Verification items for the finished model (mm, model axes). A direction names the side the tool comes from. Give positions to 0.01 mm unless a question says otherwise; leave off trailing zeros. Write each loop counter-clockwise with the first axis right and the second up, starting at its lowest first coordinate (ties: lowest second). Pieces come first, ordered by that corner, then holes. Notation, with made-up numbers: (-13.75, 69.5) -> (-7.75, 69.5) arc R33 cw to (-7.75, 107.5) -> close; hole circle Ø11 at (72.5, 82.25). An arc over 180 degrees is marked (long way). Write item = value, one per line.
from build123d import *

# Parameters (mm, degrees)
BOSS_EXTRUDE1_DEPTH = 12.7
BOSS_EXTRUDE3_DEPTH = 12.7
CUT_EXTRUDE1_REACH  = 14.7
CUT_EXTRUDE2_REACH  = 14.7
SKETCH6_W           = 7.112
SKETCH6_H           = 3.302
BOSS_EXTRUDE4_DEPTH = 3.175
SKETCH7_W           = 7.112
SKETCH7_H           = 3.302
BOSS_EXTRUDE5_DEPTH = 3.175
CUT_EXTRUDE3_REACH  = 14.7
SKETCH8_W           = 7.112
SKETCH8_H           = 3.302
CUT_EXTRUDE4_REACH  = 14.7
SKETCH9_W           = 7.112
SKETCH9_H           = 3.302


with BuildPart() as part:
    # Sketch1 → Boss-Extrude1 (new body)
    with BuildSketch(Plane(origin=(0, 0, 0), x_dir=(0, 0, -1), z_dir=(1, 0, 0))):
        Polygon((0, 0), (80.01, 0), (80.01, 19.05), (71.12, 19.05), (71.12, 8.89), (8.89, 8.89), (8.89, 19.05), (0, 19.05), align=None)
    extrude(amount=BOSS_EXTRUDE1_DEPTH)

    # Sketch2 → Boss-Extrude3 (add)
    with BuildSketch(Plane.ZY):
        Polygon((-63.5, 12.192), (-70.612, 12.192), (-70.612, 8.89), (-74.93, 8.89), (-74.93, 15.494), (-63.5, 15.494), align=None)
        Polygon((-16.51, 12.192), (-9.398, 12.192), (-9.398, 8.89), (-5.08, 8.89), (-5.08, 15.494), (-16.51, 15.494), align=None)
    extrude(amount=-BOSS_EXTRUDE3_DEPTH)

    # Sketch4 → Cut-Extrude1 (cut, up to next)
    with BuildSketch(Plane.ZY, mode=Mode.PRIVATE) as cut_extrude1_sk1:
        Polygon((-71.12, 15.494), (-75.438, 15.494), (-75.438, 0), (-80.01, 0), (-80.01, 19.05), (-71.12, 19.05), align=None)
    cut_extrude1_tool1 = extrude(cut_extrude1_sk1.sketch, amount=-CUT_EXTRUDE1_REACH, mode=Mode.PRIVATE) & part.part
    add(cut_extrude1_tool1.solids().sort_by_distance((0, 10.686074, -77.05781))[0], mode=Mode.SUBTRACT)

    # Sketch5 → Cut-Extrude2 (cut, up to next)
    with BuildSketch(Plane.ZY, mode=Mode.PRIVATE) as cut_extrude2_sk1:
        Polygon((-8.89, 15.494), (-4.572, 15.494), (-4.572, 0), (0, 0), (0, 19.05), (-8.89, 19.05), align=None)
    cut_extrude2_tool1 = extrude(cut_extrude2_sk1.sketch, amount=-CUT_EXTRUDE2_REACH, mode=Mode.PRIVATE) & part.part
    add(cut_extrude2_tool1.solids().sort_by_distance((0, 10.686074, -2.95219))[0], mode=Mode.SUBTRACT)

    # Sketch6 → Boss-Extrude4 (add)
    with BuildSketch(Plane(origin=(12.7, 0, 0), x_dir=(0, 0, -1), z_dir=(1, 0, 0))):
        with Locations((12.954, 10.541)):
            Rectangle(SKETCH6_W, SKETCH6_H)
    extrude(amount=-BOSS_EXTRUDE4_DEPTH)

    # Sketch7 → Boss-Extrude5 (add)
    with BuildSketch(Plane(origin=(12.7, 0, 0), x_dir=(0, 0, -1), z_dir=(1, 0, 0))):
        with Locations((67.056, 10.541)):
            Rectangle(SKETCH7_W, SKETCH7_H)
    extrude(amount=-BOSS_EXTRUDE5_DEPTH)

    # Sketch8 → Cut-Extrude3 (cut, up to next)
    with BuildSketch(Plane(origin=(12.7, 0, 0), x_dir=(0, 0, -1), z_dir=(1, 0, 0)), mode=Mode.PRIVATE) as cut_extrude3_sk1:
        with Locations((12.954, 10.541)):
            Rectangle(SKETCH8_W, SKETCH8_H)
    cut_extrude3_tool1 = extrude(cut_extrude3_sk1.sketch, amount=-CUT_EXTRUDE3_REACH, mode=Mode.PRIVATE) & part.part
    add(cut_extrude3_tool1.solids().sort_by_distance((12.7, 10.541, -12.954))[0], mode=Mode.SUBTRACT)

    # Sketch9 → Cut-Extrude4 (cut, up to next)
    with BuildSketch(Plane(origin=(12.7, 0, 0), x_dir=(0, 0, -1), z_dir=(1, 0, 0)), mode=Mode.PRIVATE) as cut_extrude4_sk1:
        with Locations((67.056, 10.541)):
            Rectangle(SKETCH9_W, SKETCH9_H)
    cut_extrude4_tool1 = extrude(cut_extrude4_sk1.sketch, amount=-CUT_EXTRUDE4_REACH, mode=Mode.PRIVATE) & part.part
    add(cut_extrude4_tool1.solids().sort_by_distance((12.7, 10.541, -67.056))[0], mode=Mode.SUBTRACT)


solid = part.part
Item 1: Sectioned sample at A-A on y = 10.25. Record the cut outline in (x, z), then the cut area to 3 significant figures.
Response values:
outline = (0, -75.44) -> (12.7, -75.44) -> (12.7, -70.61) -> (0, -70.61) -> close; (0, -9.4) -> (12.7, -9.4) -> (12.7, -4.57) -> (0, -4.57) -> close
area = 123 mm^2
Item 2: Mould release check, pull along Y, two halves, no side actions. Record for faces 4 (the flat face through (12.7, 6, -40)), 5 (the flat face through (6, 15.494, -70)), 6 (the flat face through (6, 8.89, -40)): +Y half, -Y half, draft (parallel to the pull), parting line (faces both ways), or undercut.
Response values:
face_4 = draft
face_5 = +Y half
face_6 = undercut
Item 3: Material ranges on line 1 (Z direction, x = 7.5, y = 14.25); line 2 (Z direction, x = 4.5, y = 11); line 3 (Y direction, x = 5.75, z = -14.5), recorded low to high.
Response values:
line_1 = -75.44 to -63.5, -16.51 to -4.57
line_2 = -75.44 to -70.61, -9.4 to -4.57
line_3 = 0 to 8.89, 12.19 to 15.49
Item 4: Go/stop test with flat-tipped pins: P1, Ø2, axis at x = 7, z = -31, coming from the -Y side; P2, Ø2, axis at x = 6.5, z = -34, coming from the +Y side. Record where each tip stops, or that it passes through.
Response values:
P1 = 0
P2 = 8.89
Item 5: Sectioned sample at C-C on x = 9. Record the cut outline in (y, z), then the cut area to 3 significant figures.
Response values:
outline = (0, -75.44) -> (15.49, -75.44) -> (15.49, -63.5) -> (12.19, -63.5) -> (12.19, -70.61) -> (8.89, -70.61) -> (8.89, -9.4) -> (12.19, -9.4) -> (12.19, -16.51) -> (15.49, -16.51) -> (15.49, -4.57) -> (0, -4.57) -> close
area = 741 mm^2
Item 6: Sectioned sample at D-D on z = -57.5. Record the cut outline in (x, y), then the cut area to 3 significant figures.
Response values:
outline = (0, 0) -> (12.7, 0) -> (12.7, 8.89) -> (0, 8.89) -> close
area = 113 mm^2
Item 7: Set-up check for faces 1 (the flat face through (6, 12.192, -13)), 2 (the flat face through (6, 14, -63.5)), 3 (the flat face through (6, 8, -4.572)): record each of +Z, -Z, +X, -X, +Y, -Y from which the full face is reachable in a straight line by a thin tool's end or side.
Response values:
face_1 = +X, -X
face_2 = +X, -X, +Y
face_3 = +Z, +X, -X, +Y, -Y
Item 8: Sectioned sample at B-B on z = -67.5. Record the cut outline in (x, y), then the cut area to 3 significant figures.
Response values:
outline = (0, 0) -> (12.7, 0) -> (12.7, 8.89) -> (0, 8.89) -> close; (0, 12.19) -> (12.7, 12.19) -> (12.7, 15.49) -> (0, 15.49) -> close
area = 155 mm^2
